Geometry: see drawing. Coordinates: mm, zero at the bounding-box minimum. Round coordinates to 2 decimals unless told otherwise and drop trailing zeros. Order: outer loops, then holes, each group sorted by start corner. A loop starts at its lowest first (then second) coordinate and runs counter-clockwise, first axis right, second up. Notation, with made-up numbers: M 87,71 L 109,71 A15 ccw 109,92 Z; hole C 35.5,-33 d2. An arc over 180 degrees is marked long. Answer in a Markdown table with one row per item. Add a question column.
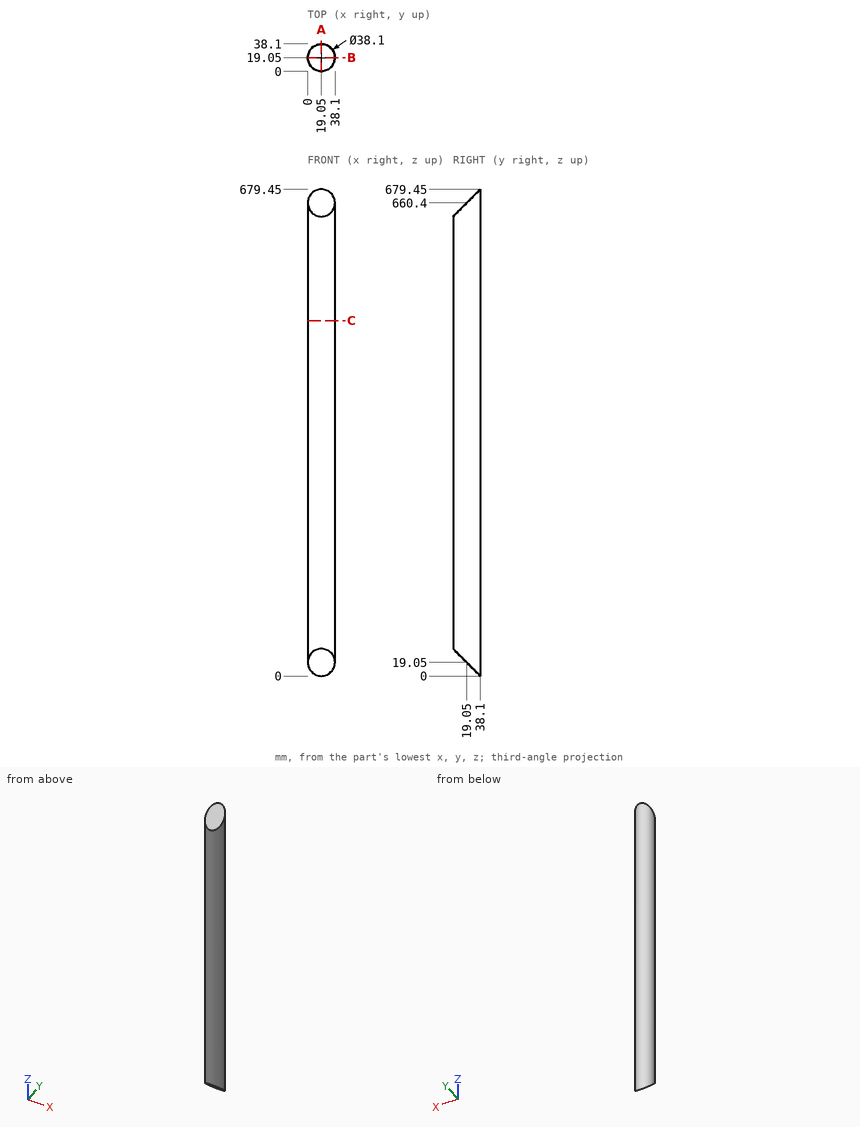
(1) Cut plane B-B (y = 19.05). Return loops of the section in (x, z).
(2) Cut plane A-A (x = 19.05). Return loops of the section in (y, z), and give its area (3 significant figures).
(3) Cut plane C-C (z = 496). Return loops of the section in (x, y).
(4) Pin query (flat end, axial travel): pin 1 (5 mm diameter, centred on x = 29, z = 376, fed in from +Y); pin 2 (8 mm diameter, centred on y = 10.5, z = 371, fed in from -X); pin 3 (2 mm diameter, centred on y = 29.5, z = 377, fed in from -X). Return the tip coordinate at first contact, or that it passes through.
(5) Line query: line 1 (Y direction, x = 17.5, z = 325); line 2 (X direction, y = 19.5, z = 248.5); line 3 (Y direction, x = 22, z = 627). Output: solid intervals per line, ascending. Write a range as from..to.
Answer list:
| question | item | result |
|---|---|---|
| 1 | outline | M 0,19.05 L 38.1,19.05 L 38.1,660.4 L 0,660.4 Z |
| 2 | outline | M 0,38.1 L 38.1,0 L 38.1,679.45 L 0,641.35 Z |
| 2 | area | 24,400 mm² |
| 3 | outline | C 19.05,19.05 d38.1 |
| 4 | pin 1 | y = 36.58 |
| 4 | pin 2 | x = 0.55 |
| 4 | pin 3 | x = 2.51 |
| 5 | line 1 | 0.06..38.04 |
| 5 | line 2 | 0.01..38.09 |
| 5 | line 3 | 0.23..37.87 |
